Autodesk Inventor part; units mm, degrees
ref_plane "Work Plane1" through (440.1475, 57.8945, 0) normal (-0.9848, 0.1736, 0) x (0, 0, 1)
ref_plane "YZ Plane" through (0, 0, 0) normal (1, 0, 0) x (0, 1, 0)
ref_plane "XZ Plane" through (0, 0, 0) normal (0, 1, 0) x (-1, 0, 0)
sketch "Sketch1" plane through (0, 0, 0) normal (0, 0, 1) x (1, 0, 0)
  ellipse E0 centre (0, 0) end of major axis (0, 330) minor radius 450 (0, -330) -> (0, 330) ccw
  ellipse E1 centre (0, 0) end of major axis (420, 0) minor radius 300 (0, -300) -> (0, 300) ccw
  line L0 (0, 300) -> (0, 330)
  line L1 (0, -300) -> (0, -330)
  line L2 (420, 0) -> (450, 0)
  dimension "d0" = 420
  dimension "d1" = 450
  dimension "d2" = 300
  dimension "d3" = 330
extrude "Extrusion1" add sketch "Sketch1" along normal blind 80
sketch "Sketch2" plane through (0, 0, 80) normal (0, 0, 1) x (1, 0, 0)
  line L0 (0, 0) -> (451.5059, 0)
  ellipse E0 centre (0, 0) end of major axis (-450, 0) minor radius 330 (0, -330) -> (0, 330) ccw
  line L1 (0, 330) -> (0, 300)
  ellipse E1 centre (0, 0) end of major axis (-420, 0) minor radius 300 (0, -300) -> (0, 300) ccw
  line L2 (0, -300) -> (0, -330)
  point P0 (420, 0)
  point P1 (450, 0)
revolve "Revolution1" add sketch "Sketch2" angle 180 about axis through (0, 0, 80) along (1, 0, 0) contours E1 L1 E0 L0
sketch "Sketch3" plane through (0, 0, 0) normal (0, 0, -1) x (-1, 0, 0)
  ellipse E0 centre (0, 0) end of major axis (420, 0) minor radius 300 (0, 300) -> (0, -300) ccw
  line L0 (-410.6033, 63.104) -> (-375.8737, -133.8576)
  line L1 (-375.8737, -133.8576) -> (-428.5073, -143.1383)
  line L2 (-428.5073, -143.1383) -> (-456.291, 14.4309)
  line L3 (0, 300) -> (0, -300)
  ellipse E1 centre (0, 0) end of major axis (450, 0) minor radius 330 (0, 330) -> (0, -330) ccw
  line L4 (-456.291, 14.4309) -> (-439.6592, 70.3382)
  line L5 (-428.5073, -143.1383) -> (-336.4493, -219.1451)
  line L6 (-336.4493, -219.1451) -> (-375.8737, -133.8576)
  line L7 (-410.6033, 63.104) -> (-439.6592, 70.3382)
  line L8 (-393.2385, -35.3768) -> (260.9914, 90.2506)
  line L9 (260.9914, 90.2506) -> (260.9914, 44.7879)
  line L10 (260.9914, 44.7879) -> (0, 40.1342)
  dimension "d8" = 200
  dimension "d9" = 10
  dimension "d12" = 45.4627
  dimension "d13" = 160
extrude "Extrusion2" add sketch "Sketch3" against normal blind 160 contours L0 E0
ref_plane "Work Plane1" through (440.1475, 57.8945, 0) normal (-0.9848, 0.1736, 0) x (0, 0, 1)
sketch "Sketch5" plane through (440.1475, 57.8945, 0) normal (-0.9848, 0.1736, 0) x (0, 0, 1)
  line L0 (80, -458.4323) -> (80, -55.3041)
  circle A0 centre (80, -117.2866) radius 241.1725
  point P0 (0, -133.4458)
extrude "Extrusion4" cut sketch "Sketch5" against normal blind 160
sketch "Sketch6" plane through (0, -330, 0) normal (-1, 0, 0) x (0, 0, 1)
  line L0 (0, 30) -> (0, 0)
  line L1 (0, 0) -> (80, 0)
  arc A0 (80, 0) -> (80, 660) centre (80, 330) ccw
  line L2 (0, 660) -> (80, 660)
  line L3 (0, 660) -> (0, 630)
  line L4 (0, 630) -> (80, 630)
  arc A1 (80, 30) -> (80, 630) centre (80, 330) ccw
  line L5 (0, 30) -> (80, 30)
  arc A2 (80, -50) -> (80, 710) centre (80, 330) ccw
  line L6 (80, -50) -> (-50, -50)
  line L7 (-50, -50) -> (-50, 80)
  line L8 (-50, 80) -> (80, 80)
  arc A3 (80, 80) -> (80, 580) centre (80, 330) ccw
  line L9 (80, 580) -> (-50, 580)
  line L10 (-50, 580) -> (-50, 710)
  line L11 (-50, 710) -> (80, 710)
  line L12 (0, 660) -> (0, 710)
  line L13 (0, 0) -> (0, -50)
  line L14 (80, 330) -> (410, 330)
  circle A4 centre (435, 330) radius 4.25
  circle A5 centre (426.0994, 408.9949) radius 4.25
  circle A6 centre (399.844, 484.0287) radius 4.25
  circle A7 centre (357.5502, 551.3389) radius 4.25
  circle A8 centre (301.3389, 607.5502) radius 4.25
  circle A9 centre (234.0288, 649.8439) radius 4.25
  circle A10 centre (158.995, 676.0994) radius 4.25
  circle A11 centre (80, 685) radius 4.25
  circle A12 centre (435, 330) radius 4.25
  circle A13 centre (426.0994, 251.0051) radius 4.25
  circle A14 centre (399.844, 175.9713) radius 4.25
  circle A15 centre (357.5502, 108.6611) radius 4.25
  circle A16 centre (301.3389, 52.4498) radius 4.25
  circle A17 centre (234.0288, 10.1561) radius 4.25
  circle A18 centre (158.995, -16.0994) radius 4.25
  circle A19 centre (80, -25) radius 4.25
  point P0 (0, 330)
  point P1 (460, 330)
  point P2 (80, -50)
  point P3 (460, 330)
  point P4 (439.25, 330)
  point P5 (430.75, 330)
  dimension "d19" = 50
  dimension "d22" = 8.5
  dimension "d25" = 90
  dimension "d27" = 25
  dimension "d28" = 0
extrude "Extrusion5" add sketch "Sketch6" against normal blind 10 contours L5 A1 L14 A0 L1 L0 | L1 A0 L2 L12 L11 A2 L6 L13 | A1 L4 L3 L2 A0 L14
sketch "Sketch7" plane through (440.1475, 57.8945, 0) normal (0.9848, -0.1736, 0) x (0, 0, -1)
  circle A0 centre (-80, -125.7359) radius 35
  circle A1 centre (-80, -70.7359) radius 4.5
  circle A2 centre (-118.8909, -86.845) radius 4.5
  circle A3 centre (-135, -125.7359) radius 4.5
  circle A4 centre (-118.8909, -164.6268) radius 4.5
  circle A5 centre (-80, -180.7359) radius 4.5
  circle A6 centre (-41.1091, -164.6268) radius 4.5
  circle A7 centre (-25, -125.7359) radius 4.5
  circle A8 centre (-41.1091, -86.845) radius 4.5
  point P0 (-80, -205.7359)
  point P1 (-80, 6.7266)
  dimension "d29" = 70
  dimension "d30" = 9
  dimension "d31" = 55
  dimension "d34" = 360
  dimension "d38" = 80
extrude "Extrusion6" cut sketch "Sketch7" against normal blind 50
properties part number "eggshellCorePrinted" material "GFRC"
Verification items for the finished model (mm, model axes). A direction names the side the tool comes from. Round coordinates to 2 decimals unless told otherwise and drop trailing zeros.
(1) Depth check by flat-ended pin: pin 1 Ø10 at (y, z) = (-78.99, 426.1) entering from +X; pin 2 Ø12 at (x, y) = (80, -30.5) entering from +Z; pin 3 Ø2 at (x, y) = (47, -174) entering from +Z; pin 4 Ø13.5 at (y, z) = (-221.34, 357.55) entering from -X. Enter the tip coordinate at first touch or a pass-through.
Returned:
pin 1: stops at x = 10
pin 2: stops at z = 404.25
pin 3: stops at z = 358.9
pin 4: stops at x = 0
(2) Access from +Z, -Z, +X, -X, +Y, -Y to the whole of each face (thin tool, end or side, straight path). Record for faces 5 (the flat face through (10, 2, 416)), 6 (the cylindrical face through (4.93, -8.36, 459.91)).
Returned:
face 5: +Z, +X
face 6: +Z, +X, -X
(3) Material ranges on line 1 (Z direction, x = 413, y = -80); line 2 (Y direction, x = 111.5, z = 186); line 3 (Y direction, x = 127.5, z = 118.5), recorded low to high.
Returned:
line 1: z = 0 to 48.27, 111.73 to 183.79
line 2: y = -301.63 to -269.11, 269.11 to 301.63
line 3: y = -314.13 to -283.24, 283.24 to 314.13
(4) Mould release check, pull along Y, two halves, no side actions. Record for faces 1 (the flat face through (0, -30, 384)), 2 (the cylindrical face through (405.573, -53.009, 46.616)), 3 (the flat face through (427.224, -15.384, 91.449)), 4 (the flat face through (397.34, -12.11, 78.88)): pulls with the +Y half, pulls with the -Y half, needs draft (parallel to the pull), parting line crosses it, or undercut.
Returned:
face 1: needs draft
face 2: undercut
face 3: pulls with the -Y half
face 4: undercut
